Verification items for this drawing (mm, ordinates from the low corner). Coordinates: 2 decimals unless noted, no trailing zeros. Order: outer loops, then holes, each group sorted by start corner. A loop starts at its lowest first (then second) coordinate and runs counter-clockwise, first axis right, second up. Notation, with made-up numbers: M 32.5,-23.75 L 43.5,-23.75 A23 cw 43.5,-9.75 Z; hole C -35,-32.5 d8. An arc over 180 degrees is marked long. Answer as a JSON object with one key per item and string values. Group by question number.
(1) Cross-section at A-A (y = 53.5). Enter the section's corners in (x, z), plus the area to 3 significant figures.
(2) Material ranges on line 1 (Z direction, x = 2.5, y = 13.5); line 2 (Z direction, x = 4.15, y = 60); line 3 (Z direction, x = 0.35, y = 24.5), recorded low to high.
(3) Cross-section at C-C (y = 21). Enter the section's corners in (x, z), plus the area to 3 significant figures.
(4) Gauge pin test, flat ends, axial feed: pin 1 Ø3 at (x, z) = (4, 85) entering from +Y; pin 2 Ø1.5 at (x, z) = (1.5, 67) entering from -Y; pin 3 Ø3 at (x, y) = (3, 59) entering from +Z; pin 4 Ø8 at (y, z) = (56.5, 17) entering from -X. Record the tip position at first contact, or that the pin passes through.
(5) Cross-section at D-D (z = 92.5). Enter the section's corners in (x, y), plus the area to 3 significant figures.
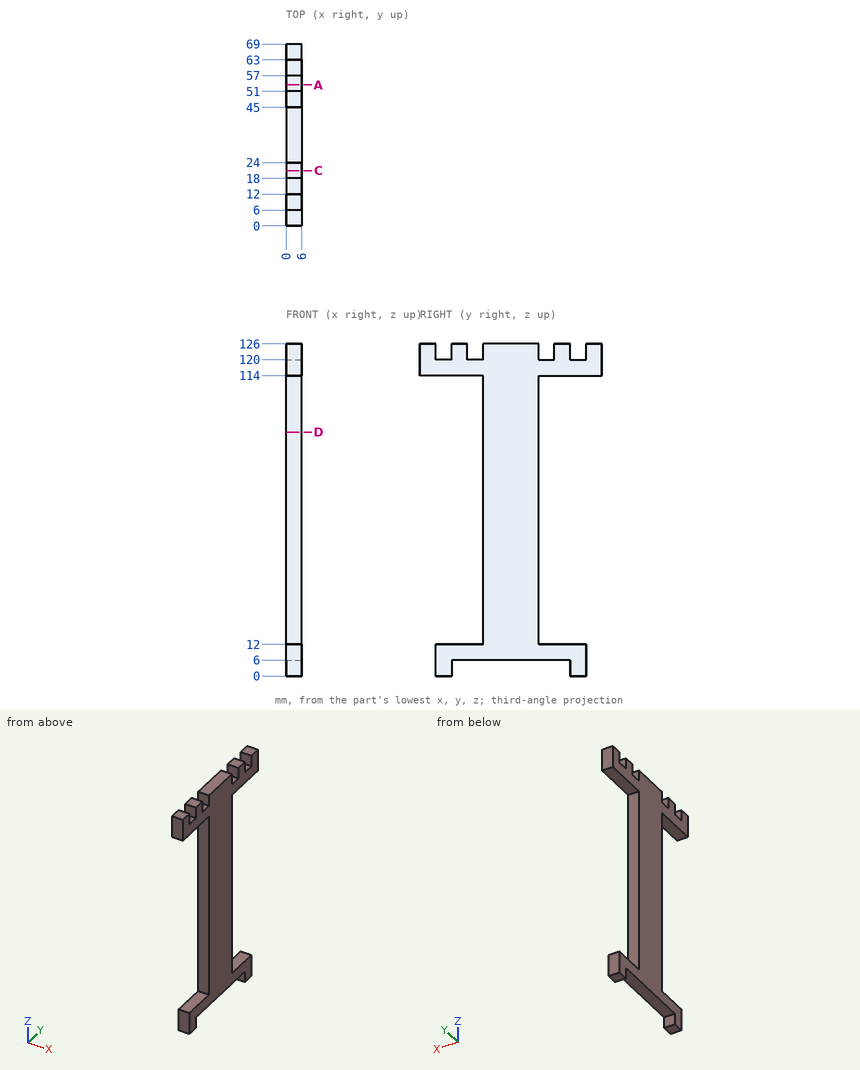
Taken from the geometry:
{
 "1": {"outline": "M 0,6 L 6,6 L 6,12 L 0,12 Z; M 0,114 L 6,114 L 6,126 L 0,126 Z", "area": "108 mm²"},
 "2": {"line 1": "z = 6 to 12, 114 to 126", "line 2": "z = 0 to 12, 114 to 120", "line 3": "z = 6 to 126"},
 "3": {"outline": "M 0,6 L 6,6 L 6,12 L 0,12 Z; M 0,114 L 6,114 L 6,120 L 0,120 Z", "area": "72.0 mm²"},
 "4": {"pin 1": "stops at y = 45", "pin 2": "stops at y = 24", "pin 3": "stops at z = 120", "pin 4": "passes through"},
 "5": {"outline": "M 0,24 L 6,24 L 6,45 L 0,45 Z", "area": "126 mm²"}
}
